from build123d import *

# Parameters (mm, degrees)
BOSS_EXTRUDE1_DEPTH = 55
BOSS_EXTRUDE2_START = 15
SKETCH2_R           = 5
SKETCH2_R_2         = 2.75
BOSS_EXTRUDE2_DEPTH = 6
CUT_EXTRUDE1_START  = 15
SKETCH2_4_R         = 2.75
CUT_EXTRUDE1_DEPTH  = 4
SKETCH3_W           = 40
SKETCH3_H           = 3
CUT_EXTRUDE2_DEPTH  = 10
BOSS_EXTRUDE3_START = 15
SKETCH2_5_R         = 2.75
BOSS_EXTRUDE3_DEPTH = 1


with BuildPart() as part:
    # Sketch1 → Boss-Extrude1 (new body)
    with BuildSketch(Plane(origin=(0, 0, 0), x_dir=(1, 0, 0), z_dir=(0, 1, 0))):
        with BuildLine():
            Line((-3, 5), (-3, 10))
            Line((-3, 10), (0, 10))
            Line((0, 10), (0, 5))
            ThreePointArc((0, 5), (1.464466094, 1.464466094), (5, 0))
            Line((5, 0), (125, 0))
            ThreePointArc((125, 0), (128.535533906, 1.464466094), (130, 5))
            Line((130, 5), (130, 10))
            Line((130, 10), (133, 10))
            Line((133, 10), (133, 5))
            ThreePointArc((133, 5), (130.656854249, -0.656854249), (125, -3))
            Line((125, -3), (5, -3))
            ThreePointArc((5, -3), (-0.656854249, -0.656854249), (-3, 5))
        make_face()
    extrude(amount=BOSS_EXTRUDE1_DEPTH)

    # Sketch2 → Boss-Extrude2 (add)
    with BuildSketch(Plane(origin=(0, 0, 0), x_dir=(1, 0, 0), z_dir=(0, 1, 0)).offset(BOSS_EXTRUDE2_START)):
        with BuildLine():
            Line((5, 10), (0, 10))
            Line((0, 10), (0, 5))
            ThreePointArc((0, 5), (1.464466094, 8.535533906), (5, 10))
        make_face()
        with Locations((5, 5)):
            Circle(SKETCH2_R)
        with Locations((5, 5)):
            Circle(SKETCH2_R_2, mode=Mode.SUBTRACT)
        with BuildLine():
            Line((10, 0), (10, 5))
            ThreePointArc((10, 5), (8.535533906, 1.464466094), (5, 0))
            Line((5, 0), (10, 0))
        make_face()
        with BuildLine():
            Line((120, 5), (120, 0))
            Line((120, 0), (125, 0))
            ThreePointArc((125, 0), (121.464466094, 1.464466094), (120, 5))
        make_face()
        with Locations((125, 5)):
            Circle(SKETCH2_R)
        with Locations((125, 5)):
            Circle(SKETCH2_R_2, mode=Mode.SUBTRACT)
        with Locations((125, 5)):
            Circle(SKETCH2_R_2)
        with BuildLine():
            ThreePointArc((125, 10), (128.535533906, 8.535533906), (130, 5))
            Line((130, 5), (130, 10))
            Line((130, 10), (125, 10))
        make_face()
        with Locations((5, 5)):
            Circle(SKETCH2_R_2)
    extrude(amount=BOSS_EXTRUDE2_DEPTH)

    # Sketch2<4> → Cut-Extrude1 (cut)
    with BuildSketch(Plane(origin=(0, 0, 0), x_dir=(1, 0, 0), z_dir=(0, 1, 0)).offset(CUT_EXTRUDE1_START)):
        with Locations((5, 5)):
            Circle(SKETCH2_4_R)
        with Locations((125, 5)):
            Circle(SKETCH2_4_R)
    extrude(amount=CUT_EXTRUDE1_DEPTH, mode=Mode.SUBTRACT)

    # Sketch3 → Cut-Extrude2 (cut)
    with BuildSketch(Plane.XY):
        with BuildLine():
            ThreePointArc((55, 40), (56.5, 38.5), (55, 37))
            Line((55, 37), (15, 37))
            ThreePointArc((15, 37), (13.5, 38.5), (15, 40))
            Line((15, 40), (55, 40))
        make_face()
        with BuildLine():
            ThreePointArc((55, 46), (56.5, 44.5), (55, 43))
            Line((55, 43), (15, 43))
            ThreePointArc((15, 43), (13.5, 44.5), (15, 46))
            Line((15, 46), (55, 46))
        make_face()
        with BuildLine():
            Line((115, 37), (75, 37))
            ThreePointArc((75, 37), (73.5, 38.5), (75, 40))
            Line((75, 40), (115, 40))
            ThreePointArc((115, 40), (116.5, 38.5), (115, 37))
        make_face()
        with BuildLine():
            Line((115, 43), (75, 43))
            ThreePointArc((75, 43), (73.5, 44.5), (75, 46))
            Line((75, 46), (115, 46))
            ThreePointArc((115, 46), (116.5, 44.5), (115, 43))
        make_face()
        with Locations((95, 50.5)):
            Rectangle(SKETCH3_W, SKETCH3_H)
        with Locations((35, 50.5)):
            Rectangle(SKETCH3_W, SKETCH3_H)
        with BuildLine():
            ThreePointArc((15, 49), (13.5, 50.5), (15, 52))
            Line((15, 52), (15, 49))
        make_face()
        with BuildLine():
            ThreePointArc((55, 52), (56.5, 50.5), (55, 49))
            Line((55, 49), (55, 52))
        make_face()
        with BuildLine():
            Line((75, 52), (75, 49))
            ThreePointArc((75, 49), (73.5, 50.5), (75, 52))
        make_face()
        with BuildLine():
            Line((115, 52), (115, 49))
            ThreePointArc((115, 49), (116.5, 50.5), (115, 52))
        make_face()
        with BuildLine():
            ThreePointArc((55, 34), (56.5, 32.5), (55, 31))
            Line((55, 31), (15, 31))
            ThreePointArc((15, 31), (13.5, 32.5), (15, 34))
            Line((15, 34), (55, 34))
        make_face()
        with BuildLine():
            Line((115, 31), (75, 31))
            ThreePointArc((75, 31), (73.5, 32.5), (75, 34))
            Line((75, 34), (115, 34))
            ThreePointArc((115, 34), (116.5, 32.5), (115, 31))
        make_face()
    extrude(amount=CUT_EXTRUDE2_DEPTH, mode=Mode.SUBTRACT)

    # Sketch2<5> → Boss-Extrude3 (add)
    with BuildSketch(Plane(origin=(0, 0, 0), x_dir=(1, 0, 0), z_dir=(0, 1, 0)).offset(BOSS_EXTRUDE3_START)):
        with Locations((5, 5)):
            Circle(SKETCH2_5_R)
        with Locations((125, 5)):
            Circle(SKETCH2_5_R)
    extrude(amount=BOSS_EXTRUDE3_DEPTH)


solid = part.part
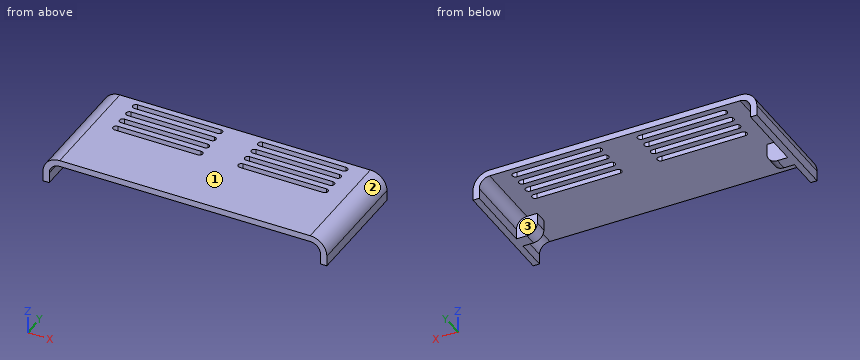
The model under review builds one solid part; all positions refer to its coordinate system, in mm. Face numbers are marked on the shaded views. Coordinates: 2 decimals unless noted, no trailing zeros. Write each loop counter-clockwise with the first axis right and the second up, starting at its lowest first coordinate (ties: lowest second). Pieces come first, ordered by that corner, then holes. Notation, with made-up numbers: (-36.75, 46) - (-17.75, 46) arc R17 cw to (-17.75, 78) - close; hole circle Ø10 at (4, 15.25). An arc over 180 degrees is marked (long way). Answer as a JSON object with one key per item and string values. Group by question number.
1. Add section A-A (y = 32.5). Give the boundary of the cut face in (x, z).
2. Clearance check with flat-ended pins moving along their axes: pin 1 Ø6 at (x, z) = (4.5, -5.5) entering from -Y; pin 2 Ø5.5 at (y, z) = (19, -2) entering from +X; pin 3 Ø1.5 at (y, z) = (19, -2.5) entering from -X. State where each tip first meets the part, or that it passes through.
3. Add section C-C (y = 24.5). Give the boundary of the cut face in (x, z), plus the area to 3 significant figures.
4. Mouldability with a two-part tool opening along X and no side actions: class the marked faces 1, 2 and 3 as pulls with the +X half, pulls with the -X half, needs draft (parallel to the pull), parting line crosses it, or undercut.
5. To check wall thickness, follow probe 1 along X at (y, z) = (16.9, -5); probe 2 along Z at (x, y) = (125, 17); probe 3 along X at (y, z) = (28.5, -4.5). State the ranges of each line that lie inside material, in increasing order.
6. Add section B-B (x = 50.5). Give the boundary of the cut face in (y, z).
Findings:
{
 "1": {"outline": "(-3, -10) - (0, -10) - (0, -5) arc R5 cw to (5, 0) - (13.5, 0) - (13.5, 3) - (5, 3) arc R8 ccw to (-3, -5) - close; (56.5, 0) - (73.5, 0) - (73.5, 3) - (56.5, 3) - close; (116.5, 0) - (125, 0) arc R5 cw to (130, -5) - (130, -10) - (133, -10) - (133, -5) arc R8 ccw to (125, 3) - (116.5, 3) - close"},
 "2": {"pin 1": "y = 15", "pin 2": "x = 133", "pin 3": "x = -2.81"},
 "3": {"outline": "(-3, -10) - (0, -10) - (0, -5) arc R5 cw to (5, 0) - (125, 0) arc R5 cw to (130, -5) - (130, -10) - (133, -10) - (133, -5) arc R8 ccw to (125, 3) - (5, 3) arc R8 ccw to (-3, -5) - close", "area": "451 mm²"},
 "4": {"face 1": "needs draft", "face 2": "pulls with the +X half", "face 3": "undercut"},
 "5": {"probe 1": "-3 to 2.25, 7.75 to 10, 120 to 122.25, 127.75 to 133", "probe 2": "-10 to -7.75, -2.25 to 3", "probe 3": "-2.98 to 0.03, 129.97 to 132.98"},
 "6": {"outline": "(0, 0) - (31, 0) - (31, 3) - (0, 3) - close; (34, 0) - (37, 0) - (37, 3) - (34, 3) - close; (40, 0) - (43, 0) - (43, 3) - (40, 3) - close; (46, 0) - (49, 0) - (49, 3) - (46, 3) - close; (52, 0) - (55, 0) - (55, 3) - (52, 3) - close"}
}
